```python
from build123d import *

# Parameters (mm, degrees)
EXTRUDE_1_DEPTH     = 300
CUT_EXTRUDE_1_DEPTH = 51


with BuildPart() as part:
    # Эскиз1 → Вытянуть-Тонкостенный1 (new body)
    with BuildSketch(Plane(origin=(0, 0, 0), x_dir=(0, 0, -1), z_dir=(1, 0, 0))):
        Polygon((0, 50), (0, 0), (50, 0), (50, 6), (6, 6), (6, 50), align=None)
    extrude(amount=EXTRUDE_1_DEPTH)

    # Эскиз2 → Вырез-Вытянуть1 (cut, through all)
    with BuildSketch(Plane.XY):
        Polygon((287.773512033, 50), (300, 50), (300, 6), align=None)
    extrude(amount=-CUT_EXTRUDE_1_DEPTH, mode=Mode.SUBTRACT)


solid = part.part
```
The listing builds one solid part. Answer for the finished solid, in the listing's coordinates (mm). A direction names the side the tool comes from. Round coordinates to 2 decimals unless told otherwise and drop trailing zeros. Loops run counter-clockwise (first coordinate to the right, second up) from the corner with the lowest first, then second, coordinate; pieces in that order, holes last. Notation, with made-up numbers: (25, 29) - (58, 29) arc R23 cw to (58, 58) - close; hole circle Ø4 at (-5.75, 38). An arc over 180 degrees is marked (long way). Return JSON: item names as keys, results as strings. Group by question number.
1. The part is cut by section C-C on z = -18. Determine the outline of the cut face in (x, y).
2. The part is cut by section A-A on x = 136. Determine the outline of the cut face in (y, z), then the cut area to 3 significant figures.
3. Consider probe 1 along Y at (x, z) = (257, -11); probe 2 along Z at (x, y) = (265, 11). Determine where each line is inside the solid, lowest interval first.
4. The part is cut by section B-B on y = 33. Determine the outline of the cut face in (x, z), then the cut area to 3 significant figures.
5. Each of these flat-tipped pins is pushed along its axis until it touches: P1, Ø6, axis at x = 190.5, y = 14, coming from the -Z side; P2, Ø13, axis at x = 121, z = -37.5, coming from the +Y side. Where does it stop, or does it pass through?
6. Which of the six approach directions +Z, -Z, +X, -X, +Y, -Y give full straight-line access (tool end or side, diameter ignored) to faces 1 (the flat face through (148, 28, -6)), 2 (the flat face through (300, 3, -25))?
Resolved:
{
 "1": {"outline": "(0, 0) - (300, 0) - (300, 6) - (0, 6) - close"},
 "2": {"outline": "(0, -50) - (6, -50) - (6, -6) - (50, -6) - (50, 0) - (0, 0) - close", "area": "564 mm²"},
 "3": {"probe 1": "y = 0 to 6", "probe 2": "z = -6 to 0"},
 "4": {"outline": "(0, -6) - (292.5, -6) - (292.5, 0) - (0, 0) - close", "area": "1,750 mm²"},
 "5": {"P1": "stops at z = -6", "P2": "stops at y = 6"},
 "6": {"face 1": "-Z, +X, -X, +Y", "face 2": "+Z, -Z, +X, +Y, -Y"}
}
